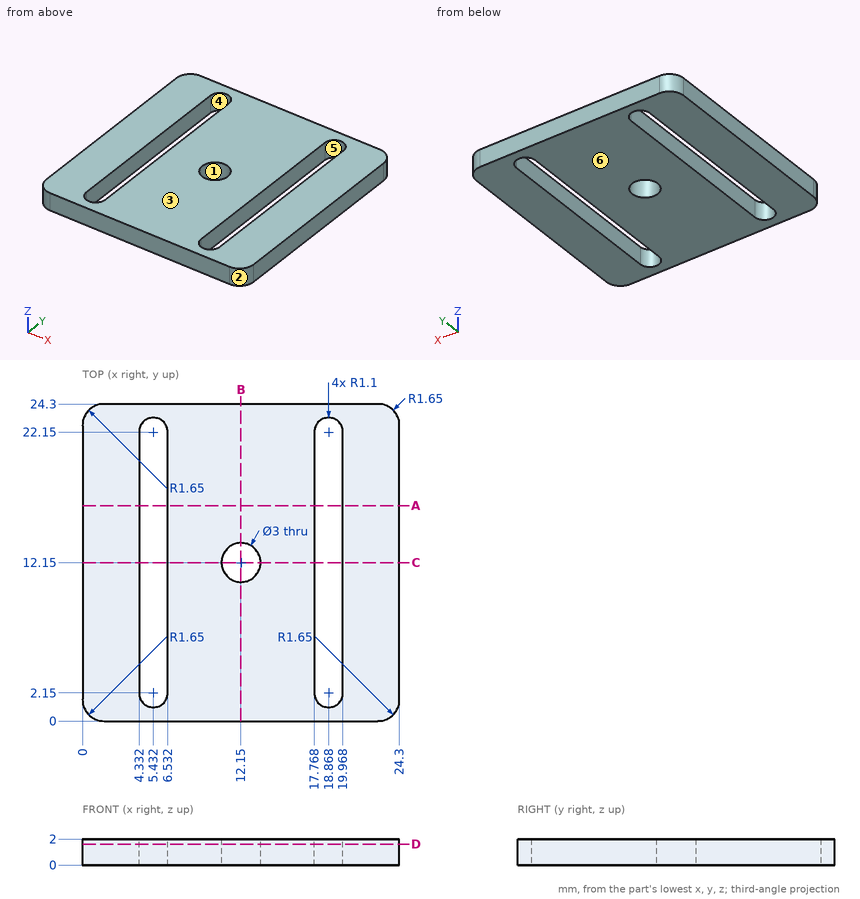
Source: three-view drawing plus pictorial views. Frame: mm from the lowest corner of the part. A direction names the side the tool comes from. Round coordinates to 2 decimals unless told otherwise and drop trailing zeros. Loops run counter-clockwise (first coordinate to the right, second up) from the corner with the lowest first, then second, coordinate; pieces in that order, holes last. Notation, with made-up numbers: M -13,38.5 L 20,38.5 A9 cw 20,51.5 Z; hole C 67.25,65 d10. An arc over 180 degrees is marked long. Answer as CSV lines item,"result". Start each with the question number.
(1) Section B-B, the plane x = 12.15. Output: boundary loops of the cut face in (y, z), plus the area to 3 significant figures.
(2) Draft query along X for the marked faces 1, 2, 3 and 4. Return one class per face: released by +X, released by -X, zero draft, split by the parting line, or undercut.
(3) Reachability of the marked faces 5 and 6 from +Z, -Z, +X, -X, +Y, -Y: full face, straight path, thin tool, end or side. Return the list, or none.
(4) Section D-D, the plane z = 1.6. Output: boundary loops of the cut face in (x, y).
(5) Section C-C, the plane y = 12.15. Output: boundary loops of the cut face in (x, z), plus the area to 3 significant figures.
(6) Line query: line 1 (X direction, y = 5.25, z = 0.3); line 2 (Y direction, x = 12.15, z = 0.8); line 3 (Y direction, x = 13.5, z = 1.75) (1 decimal). Output: solid intervals per line, ascending. Write a range as [from, to].
(7) Section A-A, the plane y = 16.5. Output: boundary loops of the cut face in (x, z).
Values found:
1,outline,"M 0,0 L 10.65,0 L 10.65,2 L 0,2 Z; M 13.65,0 L 24.3,0 L 24.3,2 L 13.65,2 Z"
1,area,"42.6 mm²"
2,face 1,"undercut"
2,face 2,"released by +X"
2,face 3,"zero draft"
2,face 4,"undercut"
3,face 5,"+Z, -Z"
3,face 6,"-Z, +X, -X, +Y, -Y"
4,outline,"M 0,1.65 A1.65 ccw 1.65,0 L 22.65,0 A1.65 ccw 24.3,1.65 L 24.3,22.65 A1.65 ccw 22.65,24.3 L 1.65,24.3 A1.65 ccw 0,22.65 Z; hole M 4.33,2.15 A1.1 ccw 6.53,2.15 L 6.53,22.15 A1.1 ccw 4.33,22.15 Z; hole C 12.15,12.15 d3; hole M 17.77,2.15 A1.1 ccw 19.97,2.15 L 19.97,22.15 A1.1 ccw 17.77,22.15 Z"
5,outline,"M 0,0 L 4.33,0 L 4.33,2 L 0,2 Z; M 6.53,0 L 10.65,0 L 10.65,2 L 6.53,2 Z; M 13.65,0 L 17.77,0 L 17.77,2 L 13.65,2 Z; M 19.97,0 L 24.3,0 L 24.3,2 L 19.97,2 Z"
5,area,"33.8 mm²"
6,line 1,"x = [0, 4.33], [6.53, 17.77], [19.97, 24.3]"
6,line 2,"y = [0, 10.65], [13.65, 24.3]"
6,line 3,"y = [0, 11.5], [12.8, 24.3]"
7,outline,"M 0,0 L 4.33,0 L 4.33,2 L 0,2 Z; M 6.53,0 L 17.77,0 L 17.77,2 L 6.53,2 Z; M 19.97,0 L 24.3,0 L 24.3,2 L 19.97,2 Z"
